Model file for the job. Use its own axes, mm. Face numbers are marked on the shaded views. A direction names the side the tool comes from. Round coordinates to 2 decimals unless told otherwise and drop trailing zeros. Order: outer loops, then holes, each group sorted by start corner. A loop starts at its lowest first (then second) coordinate and runs counter-clockwise, first axis right, second up. Notation, with made-up numbers: (-28, 31.25) - (25, 31.25) arc R27 ccw to (25, 53.25) - close; hole circle Ø9 at (-23.75, 8.25). An arc over 180 degrees is marked (long way). Put each result on its own line as item: value. Start each with the question number.
Item 1: Mould opens along Y. For the marked faces 1, 2, 3 and 4 say: pulls with the +Y half, pulls with the -Y half, needs draft (parallel to the pull), parting line crosses it, or undercut.
Item 2: Saw through at B-B on y = -7. List the corners of the cut face in (x, z), plus the area to 3 significant figures.
Item 3: Saw through at D-D on x = 23. List the corners of the cut face in (y, z).
Item 4: Pin check, flat tips, straight feed: pin 1 Ø8 at (x, z) = (23, 7.5) entering from +Y; pin 2 Ø6 at (x, z) = (-37, 14.5) entering from -Y; pin 3 Ø10 at (x, z) = (24.5, 8.5) entering from -Y; pin 4 Ø17.5 at (x, y) = (-43, -4) entering from +Z. Stop position of each tip, or through.
Item 5: Which spindle directions (+Z, -Z, +X, -X, +Y, -Y) get a long thin tool onto all of the face, cutting with end or side? Do the marked faces 5, 6, 7 and 8. Say none if no direction does.
Item 6: Probe probe 1 along Y at (x, z) = (28, 18.5); probe 2 along Y at (x, z) = (0, 6.5); probe 3 along X at (y, z) = (9, 8) (3 decimals). List the from-to ranges inside material, lowest first.
Item 7: Saw through at C-C on y = 0. List the corners of the cut face in (x, z), plus the area to 3 significant figures.
Item 8: Saw through at A-A on x = -49. List the corners of the cut face in (y, z), plus the area to 3 significant figures.
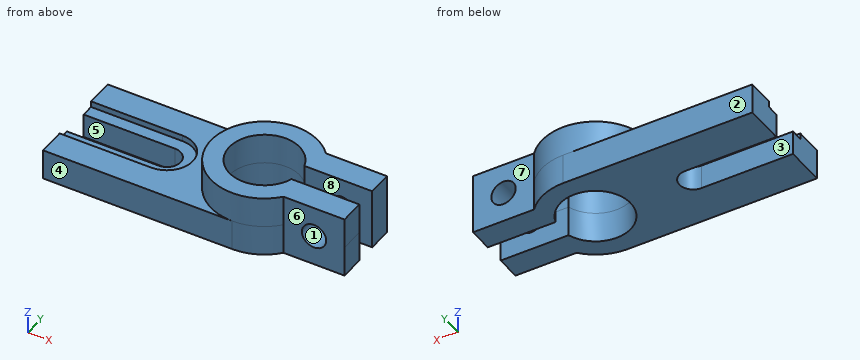
```python
from build123d import *

# Parameters (mm, degrees)
BOSS_EXTRU_1_DEPTH      = 10
BOSS_EXTRU_2_DEPTH      = 10
ENL_V_START             = -2
ENL_V_MAT_EXTRU_1_DEPTH = 2
ESQUISSE4_R             = 4
ENL_V_MAT_EXTRU_2_DEPTH = 72.309185944


with BuildPart() as part:
    # Esquisse1 → Boss.-Extru.1 (new body)
    with BuildSketch(Plane.XY):
        with BuildLine():
            Line((-62, 17.5), (-62, 4.5))
            Line((-62, 4.5), (-32, 4.5))
            ThreePointArc((-32, 4.5), (-27.5, 0), (-32, -4.5))
            Line((-32, -4.5), (-62, -4.5))
            Line((-62, -4.5), (-62, -17.5))
            Line((-62, -17.5), (0, -17.5))
            ThreePointArc((0, -17.5), (7.245688373, -15.929532322), (13.190905958, -11.5))
            Line((13.190905958, -11.5), (33.190905958, -11.5))
            Line((33.190905958, -11.5), (33.190905958, -3.5))
            Line((33.190905958, -3.5), (10.95445115, -3.5))
            ThreePointArc((10.95445115, -3.5), (-11.5, 0), (10.95445115, 3.5))
            Line((10.95445115, 3.5), (33.190905958, 3.5))
            Line((33.190905958, 3.5), (33.190905958, 11.5))
            Line((33.190905958, 11.5), (13.190905958, 11.5))
            ThreePointArc((13.190905958, 11.5), (7.245688373, 15.929532322), (0, 17.5))
            Line((0, 17.5), (-62, 17.5))
        make_face()
    extrude(amount=BOSS_EXTRU_1_DEPTH)

    # Esquisse2 → Boss.-Extru.2 (add)
    with BuildSketch(Plane.XY.offset(10)):
        with BuildLine():
            Line((13.190905958, 11.5), (33.190905958, 11.5))
            Line((33.190905958, 11.5), (33.190905958, 3.5))
            Line((33.190905958, 3.5), (10.95445115, 3.5))
            ThreePointArc((10.95445115, 3.5), (-11.5, 0), (10.95445115, -3.5))
            Line((10.95445115, -3.5), (33.190905958, -3.5))
            Line((33.190905958, -3.5), (33.190905958, -11.5))
            Line((33.190905958, -11.5), (13.190905958, -11.5))
            ThreePointArc((13.190905958, -11.5), (-17.5, 0), (13.190905958, 11.5))
        make_face()
    extrude(amount=BOSS_EXTRU_2_DEPTH)

    # Esquisse3 → Enlèv. mat.-Extru.1 (cut)
    with BuildSketch(Plane.XY.offset(10).offset(ENL_V_START)):
        with BuildLine():
            Line((-32, 4.5), (-62, 4.5))
            Line((-62, 4.5), (-62, 8.5))
            Line((-62, 8.5), (-32, 8.5))
            ThreePointArc((-32, 8.5), (-23.5, 0), (-32, -8.5))
            Line((-32, -8.5), (-62, -8.5))
            Line((-62, -8.5), (-62, -4.5))
            Line((-62, -4.5), (-32, -4.5))
            ThreePointArc((-32, -4.5), (-27.5, 0), (-32, 4.5))
        make_face()
    extrude(amount=ENL_V_MAT_EXTRU_1_DEPTH, mode=Mode.SUBTRACT)

    # Esquisse4 → Enlèv. mat.-Extru.2 (cut, through all)
    with BuildSketch(Plane.XZ.offset(11.5)):
        with Locations((23.190905958, 10)):
            Circle(ESQUISSE4_R)
    extrude(amount=-ENL_V_MAT_EXTRU_2_DEPTH, mode=Mode.SUBTRACT)


solid = part.part
```
Results found:
1. face 1: needs draft
1. face 2: pulls with the +Y half
1. face 3: undercut
1. face 4: pulls with the -Y half
2. outline: (-62, 0) - (-9.12, 0) - (-9.12, 20) - (-16.04, 20) - (-16.04, 10) - (-27.18, 10) - (-27.18, 8) - (-62, 8) - close; (9.12, 0) - (33.19, 0) - (33.19, 20) - (9.12, 20) - close; hole circle Ø8 at (23.19, 10)
2. area: 959 mm²
3. outline: (-11.5, 0) - (-3.5, 0) - (-3.5, 6) - (-11.5, 6) - close; (-11.5, 14) - (-3.5, 14) - (-3.5, 20) - (-11.5, 20) - close; (3.5, 0) - (11.5, 0) - (11.5, 6) - (3.5, 6) - close; (3.5, 14) - (11.5, 14) - (11.5, 20) - (3.5, 20) - close
4. pin 1: stops at y = 11.5
4. pin 2: passes through
4. pin 3: stops at y = -11.5
4. pin 4: stops at z = 10
5. face 5: +Z, -Z, -X
5. face 6: +Z, -Z, +X, -Y
5. face 7: +Z, -Z, +X, +Y
5. face 8: +Z, -Z, +X
6. probe 1: y = -11.5 to -3.5, 3.5 to 11.5
6. probe 2: y = -17.5 to -11.5, 11.5 to 17.5
6. probe 3: x = -62 to -7.159, 7.159 to 19.727, 26.655 to 33.191
7. outline: (-27.5, 0) - (-11.5, 0) - (-11.5, 20) - (-17.5, 20) - (-17.5, 10) - (-23.5, 10) - (-23.5, 8) - (-27.5, 8) - close
7. area: 212 mm²
8. outline: (-17.5, 0) - (-4.5, 0) - (-4.5, 8) - (-8.5, 8) - (-8.5, 10) - (-17.5, 10) - close; (4.5, 0) - (17.5, 0) - (17.5, 10) - (8.5, 10) - (8.5, 8) - (4.5, 8) - close
8. area: 244 mm²
